```python
from build123d import *

# Parameters (mm, degrees)
SKETCH_1_R          = 40
SKETCH_1_R_2        = 30.5
EXTRUDE_1_DEPTH     = 12
SKETCH_2_R          = 1.7
CUT_EXTRUDE_1_DEPTH = 12
FILLET_1_R          = 2
FILLET_2_R          = 2


with BuildPart() as part:
    # 草图1 → 凸台-拉伸1 (new body)
    with BuildSketch(Plane.XY):
        Circle(SKETCH_1_R)
        Circle(SKETCH_1_R_2, mode=Mode.SUBTRACT)
    extrude(amount=EXTRUDE_1_DEPTH)

    # 草图2 → 切除-拉伸1 (cut)
    with BuildSketch(Plane.XY.offset(12)):
        with Locations((35, 0)):
            Circle(SKETCH_2_R)
        with Locations((0, -35)):
            Circle(SKETCH_2_R)
        with Locations((-35, 0)):
            Circle(SKETCH_2_R)
        with Locations((0, 35)):
            Circle(SKETCH_2_R)
    extrude(amount=-CUT_EXTRUDE_1_DEPTH, mode=Mode.SUBTRACT)

    # 圆角1
    fillet_1_edges = [part.edges().sort_by_distance(p)[0] for p in [
        (-30.5, 0, 12),
    ]]
    fillet(fillet_1_edges, radius=FILLET_1_R)

    # 圆角2
    fillet_2_edges = [part.edges().sort_by_distance(p)[0] for p in [
        (-40, 0, 12),
    ]]
    fillet(fillet_2_edges, radius=FILLET_2_R)


solid = part.part
```
Build history of the part. All positions in model axes, mm. Round coordinates to 2 decimals unless told otherwise and drop trailing zeros. Order: outer loops, then holes, each group sorted by start corner. A loop starts at its lowest first (then second) coordinate and runs counter-clockwise, first axis right, second up. Notation, with made-up numbers: (36, 81) - (85, 81) arc R24 ccw to (85, 120) - close; hole circle Ø3 at (-18, 26.25). An arc over 180 degrees is marked (long way). Use a Markdown table: item, result.
1) Pull direction X, two halves, no side cores. Call faces 1 (the face through (-0.37, -36.66, 6.08)), 2 (the face through (-8.67, -39.05, 4.93)), 3 (the face through (-0.37, 33.34, 6.08)), 4 (the face through (11, 31, 12)): pulls with the +X half, pulls with the -X half, needs draft (parallel to the pull), parting line crosses it, or undercut.
Recorded:
| item | result |
|---|---|
| face 1 | undercut |
| face 2 | parting line crosses it |
| face 3 | undercut |
| face 4 | needs draft |
2) Saw through at A-A on y = 0. Write the cut outline in (x, z), and give its area (3 significant figures).
Recorded:
| item | result |
|---|---|
| outline | (-40, 0) - (-36.7, 0) - (-36.7, 12) - (-38, 12) arc R2 ccw to (-40, 10) - close; (-33.3, 0) - (-30.5, 0) - (-30.5, 10) arc R2 ccw to (-32.5, 12) - (-33.3, 12) - close; (30.5, 0) - (33.3, 0) - (33.3, 12) - (32.5, 12) arc R2 ccw to (30.5, 10) - close; (36.7, 0) - (40, 0) - (40, 10) arc R2 ccw to (38, 12) - (36.7, 12) - close |
| area | 143 mm² |
3) Wall check: L1, parallel to Y at x = 0, z = 9.25; L2, parallel to Y at x = 1, z = 7; L3, parallel to X at y = 22, z = 6. Give the ranges that are in metal, low to high.
Recorded:
| item | result |
|---|---|
| L1 | y = -40 to -36.7, -33.3 to -30.5, 30.5 to 33.3, 36.7 to 40 |
| L2 | y = -39.99 to -36.37, -33.63 to -30.48, 30.48 to 33.63, 36.37 to 39.99 |
| L3 | x = -33.41 to -21.12, 21.12 to 33.41 |
4) Flat gauge pins, fed straight in: pin 1 Ø6 at (y, z) = (-21, 3.5) entering from -X; pin 2 Ø2 at (x, y) = (35, 0) entering from -Z; pin 3 Ø4 at (y, z) = (6, 5) entering from -X; pin 4 Ø3 at (x, z) = (23, 7) entering from +Y. Where does each tip first touch, or does it go through?
Recorded:
| item | result |
|---|---|
| pin 1 | stops at x = -35.72 |
| pin 2 | passes through |
| pin 3 | stops at x = -39.8 |
| pin 4 | stops at y = 33.73 |
5) Saw through at C-C on z = 7.25. Write the cut outline in (x, y).
Recorded:
| item | result |
|---|---|
| outline | circle Ø80 at (0, 0); hole circle Ø3.4 at (-35, 0); hole circle Ø61 at (0, 0); hole circle Ø3.4 at (0, -35); hole circle Ø3.4 at (0, 35); hole circle Ø3.4 at (35, 0) |
